Autodesk Inventor part; units mm, degrees
ref_plane "YZ Plane" through (0, 0, 0) normal (1, 0, 0) x (0, 1, 0)
ref_plane "XZ Plane" through (0, 0, 0) normal (0, 1, 0) x (-1, 0, 0)
ref_plane "XY Plane" through (0, 0, 0) normal (0, 0, 1) x (1, 0, 0)
sketch "Sketch1" plane through (0, 0, 0) normal (0, 1, 0) x (-1, 0, 0)
  line L0 (100, -400) -> (-100, -400)
  line L1 (-100, -400) -> (-100, -110)
  line L2 (-100, -110) -> (100, -110)
  line L3 (100, -400) -> (100, -110)
  line L4 (100, -110) -> (100, -400)
  line L5 (-100, -90) -> (100, -90)
  line L6 (100, -110) -> (100, -90)
  line L7 (-100, -110) -> (-100, -90)
  line L8 (-80, -390) -> (-80, -110)
  line L9 (80, -390) -> (80, -110)
  line L10 (-80, -380) -> (80, -380)
  point P0 (0, -100)
  point P1 (90, -100)
  point P2 (-90, -100)
  dimension "d126" = 160
  dimension "d160" = 290
extrude "Extrusion1" add sketch "Sketch1" along normal blind 10 contours L0 L1 L2 L8 L10 L9 L3 | L2 L7 L5 L6
sketch "Sketch12" plane through (0, 10, 0) normal (0, 1, 0) x (1, 0, 0)
  line L0 (90, 400) -> (90, 320)
  line L1 (90, 320) -> (90, 250)
  line L2 (90, 250) -> (90, 180)
  point P0 (0, 0)
  dimension "d132" = 80
  dimension "d134" = 70
  dimension "d135" = 70
hole "Hole9" at (90, 10, -320) at (90, 10, -250) at (90, 10, -180) direction (0, -1, 0) diameter 3.2 end through all
pattern_linear "Rectangular Pattern1" count 2 spacing 180 along (-1, 0, 0) of "Hole9"
hole "Hole12" at (90, 0, -100) at (-90, 0, -100) direction (0, 1, 0) diameter 3.4 end through all
hole "Hole13" at (0, 0, -100) direction (0, 1, 0) diameter 3 end through all
properties part number "Aufhängung_Seitenteil_Koppeltest_außen"
Verification items for the finished model (mm, model axes). A direction names the side the tool comes from. Round coordinates to 2 decimals unless told otherwise and drop trailing zeros. Loops run counter-clockwise (first coordinate to the right, second up) from the corner with the lowest first, then second, coordinate; pieces in that order, holes last. Notation, with made-up numbers: (2, 8) -> (59, 8) arc R18 ccw to (59, 42) -> close; hole circle Ø9 at (87, 69.5). An arc over 180 degrees is marked (long way). Answer as a JSON object with one key per item and string values.
Q1. Draft check along X on faces 1 (the flat face through (80, 5, -247)), 2 (the flat face through (-100, 5, -247)), 3 (the flat face through (90, 10, -243)). Enter one of: pulls with the +X half, pulls with the -X half, needs draft (parallel to the pull), parting line crosses it, or undercut.
Data:
{"face 1": "undercut", "face 2": "pulls with the -X half", "face 3": "needs draft"}
Q2. Section check B-B (x = -63). Record the boundary of the cut face in (y, z).
Data:
{"outline": "(0, -400) -> (10, -400) -> (10, -380) -> (0, -380) -> close; (0, -110) -> (10, -110) -> (10, -90) -> (0, -90) -> close"}
Q3. Section check A-A (z = -256). Record the boundary of the cut face in (x, y).
Data:
{"outline": "(-100, 0) -> (-80, 0) -> (-80, 10) -> (-100, 10) -> close; (80, 0) -> (100, 0) -> (100, 10) -> (80, 10) -> close"}
Q4. Scan lines: line 1 (X direction, y = 2.75, z = -250); line 2 (Z direction, x = -90, y = 3.75); line 3 (X direction, y = 7, z = -201.5). Record each from-to range of solid material in increasing order. Write a range as from..to.
Data:
{"line 1": "x = -100..-91.6, -88.4..-80, 80..88.4, 91.6..100", "line 2": "z = -400..-321.6, -318.4..-251.6, -248.4..-181.6, -178.4..-101.7, -98.3..-90", "line 3": "x = -100..-80, 80..100"}
Q5. Access from +Z, -Z, +X, -X, +Y, -Y to the whole of each face (thin tool, end or side, straight path). Record for faces 4 (the flat face through (100, 5, -247)), 5 (the flat face through (-80, 5, -247)).
Data:
{"face 4": "+Z, -Z, +X, +Y, -Y", "face 5": "+Y, -Y"}
Q6. Section check C-C (y = 5). State how many separate pieces and enclosed holes the cut face has, then the cut area to 3 significant figures.
Data:
{"separate pieces": "1", "enclosed holes": "10", "area": "18,700 mm2"}
